from build123d import *

# Parameters (mm, degrees)
SKETCH_1_W          = 404
SKETCH_1_H          = 250
SKETCH_1_R          = 3.5
SKETCH_1_R_2        = 6
SKETCH_1_R_3        = 29
SKETCH_1_R_4        = 2.5
SKETCH_1_R_5        = 1.8
SKETCH_1_R_6        = 5.1
SKETCH_1_R_7        = 1.5
SKETCH_1_R_8        = 4.1
SKETCH_1_R_9        = 2.1
SKETCH_1_W_2        = 36
SKETCH_1_H_2        = 46
EXTRUDE_1_DEPTH     = 1
SKETCH_2_W          = 1
SKETCH_2_H          = 250
EXTRUDE_2_DEPTH     = 30
SKETCH_3_W          = 1
SKETCH_3_H          = 250
EXTRUDE_3_DEPTH     = 8
SKETCH_4_W          = 1
SKETCH_4_H          = 250
EXTRUDE_4_DEPTH     = 8
SKETCH_5_R          = 1.7
SKETCH_5_R_2        = 4
SKETCH_5_R_3        = 1.2
CUT_EXTRUDE_1_DEPTH = 8
CHAMFER_2_SIZE      = 1
SKETCH_6_W          = 404
SKETCH_6_H          = 1
SKETCH_6_W_2        = 403
EXTRUDE_5_DEPTH     = 30
FILLET_1_R          = 1
FILLET_2_R          = 2
SKETCH_7_W          = 39.273398561
SKETCH_7_H          = 2
CUT_EXTRUDE_2_DEPTH = 2.5
SKETCH_8_W          = 16.105327303
SKETCH_8_H          = 23.169067349
SKETCH_8_W_2        = 20.44042911
SKETCH_8_H_2        = 24.240130898
CUT_EXTRUDE_3_DEPTH = 2
SKETCH_9_W          = 1
SKETCH_9_H          = 22
EXTRUDE_6_DEPTH     = 2
SKETCH_10_R         = 2.5
SKETCH_10_R_2       = 1.2
EXTRUDE_7_DEPTH     = 1.5


with BuildPart() as part:
    # Эскиз1 → Вытянуть1 (new body)
    with BuildSketch(Plane.XY):
        Rectangle(SKETCH_1_W, SKETCH_1_H)
        with Locations((134, -4)):
            Circle(SKETCH_1_R, mode=Mode.SUBTRACT)
        with Locations((-128, -24)):
            Circle(SKETCH_1_R_2, mode=Mode.SUBTRACT)
        with Locations((-128, -90)):
            Circle(SKETCH_1_R_2, mode=Mode.SUBTRACT)
        with Locations((134, 67)):
            Circle(SKETCH_1_R_3, mode=Mode.SUBTRACT)
        with Locations((109, 92)):
            Circle(SKETCH_1_R_4, mode=Mode.SUBTRACT)
        with Locations((109, 42)):
            Circle(SKETCH_1_R_4, mode=Mode.SUBTRACT)
        with Locations((159, 42)):
            Circle(SKETCH_1_R_4, mode=Mode.SUBTRACT)
        with Locations((159, 92)):
            Circle(SKETCH_1_R_4, mode=Mode.SUBTRACT)
        with Locations((124.06636679, -9.794215326)):
            Circle(SKETCH_1_R_5, mode=Mode.SUBTRACT)
        with Locations((143.984951077, 1.705784674)):
            Circle(SKETCH_1_R_5, mode=Mode.SUBTRACT)
        with Locations((134, -81)):
            Circle(SKETCH_1_R_3, mode=Mode.SUBTRACT)
        with Locations((109, -56)):
            Circle(SKETCH_1_R_4, mode=Mode.SUBTRACT)
        with Locations((159, -56)):
            Circle(SKETCH_1_R_4, mode=Mode.SUBTRACT)
        with Locations((159, -106)):
            Circle(SKETCH_1_R_4, mode=Mode.SUBTRACT)
        with Locations((109, -106)):
            Circle(SKETCH_1_R_4, mode=Mode.SUBTRACT)
        with Locations((41, 97)):
            Circle(SKETCH_1_R_6, mode=Mode.SUBTRACT)
        with Locations((41, 89.8)):
            Circle(SKETCH_1_R_7, mode=Mode.SUBTRACT)
        with Locations((41, 62)):
            Circle(SKETCH_1_R_8, mode=Mode.SUBTRACT)
        with Locations((41, 19)):
            Circle(SKETCH_1_R, mode=Mode.SUBTRACT)
        with Locations((29.888232445, 16.03712609)):
            Circle(SKETCH_1_R_5, mode=Mode.SUBTRACT)
        with Locations((52.10452645, 21.989964127)):
            Circle(SKETCH_1_R_5, mode=Mode.SUBTRACT)
        with Locations((-188, 0)):
            Circle(SKETCH_1_R_9, mode=Mode.SUBTRACT)
        with Locations((-158, -57)):
            Rectangle(SKETCH_1_W_2, SKETCH_1_H_2, mode=Mode.SUBTRACT)
    extrude(amount=EXTRUDE_1_DEPTH)

    # Эскиз2 → Вытянуть2 (add)
    with BuildSketch(Plane.XY.offset(1)):
        with Locations((201.5, 0)):
            Rectangle(SKETCH_2_W, SKETCH_2_H)
        with Locations((-201.5, 0)):
            Rectangle(SKETCH_2_W, SKETCH_2_H)
    extrude(amount=-EXTRUDE_2_DEPTH)

    # Эскиз3 → Вытянуть3 (add)
    with BuildSketch(Plane.ZY.offset(202)):
        with Locations((-28.5, 0)):
            Rectangle(SKETCH_3_W, SKETCH_3_H)
    extrude(amount=-EXTRUDE_3_DEPTH)

    # Эскиз4 → Вытянуть4 (add)
    with BuildSketch(Plane(origin=(202, 0, 0), x_dir=(0, 0, -1), z_dir=(1, 0, 0))):
        with Locations((28.5, 0)):
            Rectangle(SKETCH_4_W, SKETCH_4_H)
    extrude(amount=-EXTRUDE_4_DEPTH)

    # Эскиз5 → Вырез-Вытянуть1 (cut)
    with BuildSketch(Plane(origin=(202, 0, 0), x_dir=(0, 0, -1), z_dir=(1, 0, 0))):
        with Locations(Location((19, -109, 0), (0, 0, 90))):
            Circle(SKETCH_5_R)
        with Locations(Location((19, 109, 0), (0, 0, 270))):
            Circle(SKETCH_5_R)
        with Locations(Location((11, 3.5, 0), (0, 0, 90))):
            Circle(SKETCH_5_R)
        with Locations(Location((11, -43.5, 0), (0, 0, 90))):
            Circle(SKETCH_5_R)
        with Locations(Location((9, 59, 0), (0, 0, 90))):
            Circle(SKETCH_5_R_2)
        with Locations(Location((9, 41, 0), (0, 0, 90))):
            Circle(SKETCH_5_R_2)
        with Locations(Location((14, 72, 0), (0, 0, 90))):
            Circle(SKETCH_5_R_3)
        with Locations(Location((14, 28, 0), (0, 0, 90))):
            Circle(SKETCH_5_R_3)
        with Locations(Location((19, -94, 0), (0, 0, 90))):
            Circle(SKETCH_5_R)
        with Locations(Location((19, 94, 0), (0, 0, 270))):
            Circle(SKETCH_5_R)
        with BuildLine():
            Line((7.135803619, 0.35129058), (15.135803619, -0.375982147))
            ThreePointArc((15.135803619, -0.375982147), (16.107633836, -0.858314525), (16.5, -1.869821957))
            Line((16.5, -1.869821957), (16.5, -38.130178043))
            ThreePointArc((16.5, -38.130178043), (16.107633836, -39.141685475), (15.135803619, -39.624017853))
            Line((15.135803619, -39.624017853), (7.135803619, -40.35129058))
            ThreePointArc((7.135803619, -40.35129058), (5.988492568, -39.965084606), (5.5, -38.85745077))
            Line((5.5, -38.85745077), (5.5, -1.14254923))
            ThreePointArc((5.5, -1.14254923), (5.988492568, -0.034915394), (7.135803619, 0.35129058))
        make_face()
    extrude(amount=-CUT_EXTRUDE_1_DEPTH, mode=Mode.SUBTRACT)

    # Фаска2
    chamfer_2_edges = [part.edges().sort_by_distance(p)[0] for p in [
        (122.26636679, -9.794215326, 1),
        (28.088232445, 16.03712609, 1),
        (50.30452645, 21.989964127, 1),
        (142.184951077, 1.705784674, 1),
    ]]
    chamfer(chamfer_2_edges, length=CHAMFER_2_SIZE - 0.0001)  # a hair under: the kernel refuses the full size

    # Эскиз6 → Вытянуть5 (add)
    with BuildSketch(Plane.XY.offset(1)):
        with Locations((0, 124.5)):
            Rectangle(SKETCH_6_W, SKETCH_6_H)
        with Locations((-0.5, -124.5)):
            Rectangle(SKETCH_6_W_2, SKETCH_6_H)
    extrude(amount=-EXTRUDE_5_DEPTH)

    # Скругление1
    fillet_1_edges = [part.edges().sort_by_distance(p)[0] for p in [
        (-201, 0, 0),
        (0, 124, 0),
        (201, 0, 0),
        (0, -124, 0),
        (201, 0, -28),
        (-201, 0, -28),
    ]]
    fillet(fillet_1_edges, radius=FILLET_1_R)

    # Скругление2
    fillet_2_edges = [part.edges().sort_by_distance(p)[0] for p in [
        (0, 125, 1),
        (-202, 0, 1),
        (0, -125, 1),
        (202, 0, 1),
        (-202, 0, -29),
        (202, 0, -29),
        (-202, 125, -14),
        (202, 125, -14),
        (-202, -125, -14),
        (202, -125, -14),
    ]]
    fillet(fillet_2_edges, radius=FILLET_2_R)

    # Эскиз7 → Вырез-Вытянуть2 (cut)
    with BuildSketch(Plane(origin=(0, 0, -29), x_dir=(-1, 0, 0), z_dir=(0, 0, -1))):
        with Locations((-204.595711045, -113)):
            Rectangle(SKETCH_7_W, SKETCH_7_H)
        with Locations((-204.595711045, 113)):
            Rectangle(SKETCH_7_W, SKETCH_7_H)
        with Locations((-204.595711045, -89)):
            Rectangle(SKETCH_7_W, SKETCH_7_H)
        with Locations((-204.595711045, 89)):
            Rectangle(SKETCH_7_W, SKETCH_7_H)
    extrude(amount=-CUT_EXTRUDE_2_DEPTH, mode=Mode.SUBTRACT)

    # Эскиз8 → Вырез-Вытянуть3 (cut)
    with BuildSketch(Plane(origin=(0, 0, -29), x_dir=(-1, 0, 0), z_dir=(0, 0, -1))):
        with Locations((-198.211121585, 101.246537182)):
            Rectangle(SKETCH_8_W, SKETCH_8_H)
        with Locations((-197.698675363, -101.007536633)):
            Rectangle(SKETCH_8_W_2, SKETCH_8_H_2)
    extrude(amount=-CUT_EXTRUDE_3_DEPTH, mode=Mode.SUBTRACT)

    # Эскиз9 → Вытянуть6 (add)
    with BuildSketch(Plane(origin=(0, 0, -27), x_dir=(-1, 0, 0), z_dir=(0, 0, -1))):
        with Locations((-201.5, 101)):
            Rectangle(SKETCH_9_W, SKETCH_9_H)
        with Locations((-201.5, -101)):
            Rectangle(SKETCH_9_W, SKETCH_9_H)
    extrude(amount=EXTRUDE_6_DEPTH)

    # Эскиз10 → Вытянуть7 (add)
    # profile 1 of 2: a face of its own
    with BuildSketch(Plane.ZY.offset(-201)):
        with Locations(Location((-14, 28, 0), (0, 0, 270))):
            Circle(SKETCH_10_R)
        with Locations(Location((-14, 28, 0), (0, 0, 90))):
            Circle(SKETCH_10_R_2, mode=Mode.SUBTRACT)
    # profile 2 of 2: a face of its own
    with BuildSketch(Plane.ZY.offset(-201)):
        with Locations(Location((-14, 72, 0), (0, 0, 270))):
            Circle(SKETCH_10_R)
        with Locations(Location((-14, 72, 0), (0, 0, 90))):
            Circle(SKETCH_10_R_2, mode=Mode.SUBTRACT)
    extrude(amount=EXTRUDE_7_DEPTH)


solid = part.part
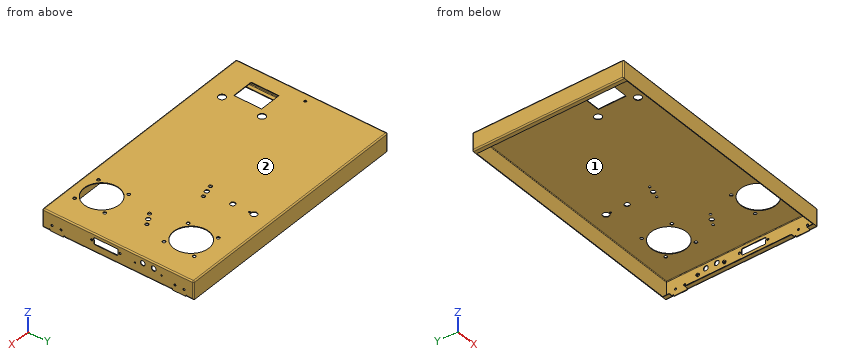
Part model, mm, in its own coordinate system. Face numbers are marked on the shaded views. Give positions to 0.01 mm unless a question says otherwise; leave off trailing zeros. Order: outer loops, then holes, each group sorted by start corner. A loop starts at its lowest first (then second) coordinate and runs counter-clockwise, first axis right, second up. Notation, with made-up numbers: (-18, -20.5) - (34, -20.5) arc R31 ccw to (34, 12.5) - close; hole circle Ø4 at (20.25, 49). An arc over 180 degrees is marked (long way). Use a Markdown table: item, result.
1) Saw through at A-A on x = -31. List the corners of the cut face in (y, z), plus the area to 3 significant figures.
Checked values:
| item | result |
|---|---|
| outline | (-125, -29) - (-124, -29) - (-124, -1) arc R1 cw to (-123, 0) - (123, 0) arc R1 cw to (124, -1) - (124, -29) - (125, -29) - (125, -1) arc R2 ccw to (123, 1) - (-123, 1) arc R2 ccw to (-125, -1) - close |
| area | 307 mm² |
2) Saw through at B-B on y = 78.5. List the corners of the cut face in (x, z), plus the area to 3 significant figures.
Checked values:
| item | result |
|---|---|
| outline | (-202, -27) arc R2 ccw to (-200, -29) - (-194, -29) - (-194, -28) - (-200, -28) arc R1 cw to (-201, -27) - (-201, -1) arc R1 cw to (-200, 0) - (107.38, 0) - (107.38, 1) - (-200, 1) arc R2 ccw to (-202, -1) - close; (160.62, 0) - (200, 0) arc R1 cw to (201, -1) - (201, -27) arc R1 cw to (200, -28) - (194, -28) - (194, -29) - (200, -29) arc R2 ccw to (202, -27) - (202, -1) arc R2 ccw to (200, 1) - (160.62, 1) - close |
| area | 420 mm² |
3) Probe L1, parallel to Y at x = 109, z = -14; L2, parallel to X at y = -69.5, z = -16.5; L3, parallel to Y at x = 134, z = 0.55. List the from-to ranges inside material, lowest first. Write a range as from..to.
Checked values:
| item | result |
|---|---|
| L1 | -125..-124, 124..125 |
| L2 | -202..-201, 201..202 |
| L3 | -124.26..-110, -52..-7.5, -0.5..38, 96..124.26 |
4) Two-plate mould, pull along X, no slides. Class the marked faces 1 and 2: +X half, -X half, draft (parallel to the pull), parting line (faces both ways), or undercut.
Checked values:
| item | result |
|---|---|
| face 1 | undercut |
| face 2 | draft |
5) Flat gauge pins, fed straight in: P1, Ø0.8, axis at x = 201.5, y = -112.5, coming from the -Z side; P2, Ø0.8, axis at x = -153, z = 0.5, coming from the +Y side; P3, Ø2.5, axis at y = -43.5, z = -11, coming from the +X side; P4, Ø14, axis at x = -128, y = -90, coming from the +Z side. Where does each tip first touch, or does it go through?
Checked values:
| item | result |
|---|---|
| P1 | z = -26.5 |
| P2 | y = 124.67 |
| P3 | x = -201 |
| P4 | z = 1 |
